Design review of the part built by this model. Coordinates are the model's own, in mm. A direction names the side the tool comes from. Give positions to 0.01 mm unless a question says otherwise; leave off trailing zeros. Loops run counter-clockwise (first coordinate to the right, second up) from the corner with the lowest first, then second, coordinate; pieces in that order, holes last. Notation, with made-up numbers: M 82.25,-10 L 91.25,-10 A18 cw 91.25,18 Z; hole C 2.5,48 d9. An arc over 180 degrees is marked long. Answer as CSV lines item,"result".
```python
from build123d import *

# Parameters (mm, degrees)
TABAN_FLAN_1_DEPTH         = 40
KES_EKSTR_ZYON1_DEPTH      = 1384.891767514
KES_EKSTR_ZYON1_DEPTH_BACK = 1384.891767514
IZIM2_W                    = 535
IZIM2_H                    = 265
KES_EKSTR_ZYON2_DEPTH      = 1384.891767514
KES_EKSTR_ZYON2_DEPTH_BACK = 1384.891767514
IZIM3_W                    = 1575
IZIM3_H                    = 360
KES_EKSTR_ZYON3_DEPTH      = 1384.891767514
KES_EKSTR_ZYON3_DEPTH_BACK = 1384.891767514
IZIM5_W                    = 535
IZIM5_H                    = 2


# Sheet-metal steps are written as plain solids
with BuildPart() as part:
    # Çizim1 → Taban-Flanş1 (new body)
    with BuildSketch(Plane.XY):
        Polygon((-517.241071282, 843.539135514), (-517.241071282, -126.460864486), (1057.758928718, -126.460864486), (1057.758928718, -891.460864486), (-1052.241071282, -891.460864486), (-1052.241071282, 843.539135514), align=None)
    extrude(amount=-TABAN_FLAN_1_DEPTH)

    # Çizim2 → Kes-Ekstrüzyon1 (cut, two sides: drawn at the far end of the back side and taken through both)
    with BuildSketch(Plane.XY.offset(-KES_EKSTR_ZYON1_DEPTH_BACK)):
        with Locations((-784.741071282, 711.039135514)):
            Rectangle(IZIM2_W, IZIM2_H)
    extrude(amount=KES_EKSTR_ZYON1_DEPTH + KES_EKSTR_ZYON1_DEPTH_BACK, mode=Mode.SUBTRACT)

    # Çizim3 → Kes-Ekstrüzyon2 (cut, two sides: drawn at the far end of the back side and taken through both)
    with BuildSketch(Plane.XY.offset(-KES_EKSTR_ZYON2_DEPTH_BACK)):
        with Locations((270.258928718, -306.460864486)):
            Rectangle(IZIM3_W, IZIM3_H)
    extrude(amount=KES_EKSTR_ZYON2_DEPTH + KES_EKSTR_ZYON2_DEPTH_BACK, mode=Mode.SUBTRACT)

    # Çizim5 → Kes-Ekstrüzyon3 (cut, two sides: drawn at the far end of the back side and taken through both)
    with BuildSketch(Plane.XY.offset(-KES_EKSTR_ZYON3_DEPTH_BACK)):
        with Locations((-784.741071282, 577.539135514)):
            Rectangle(IZIM5_W, IZIM5_H)
    extrude(amount=KES_EKSTR_ZYON3_DEPTH + KES_EKSTR_ZYON3_DEPTH_BACK, mode=Mode.SUBTRACT)


solid = part.part
```
1. We need section A-A, the plane z = -6.5. Write out the cut boundary in (x, y), plus the area to 3 significant figures.
Answer block:
outline,"M -1052.24,-891.46 L 1057.76,-891.46 L 1057.76,-486.46 L -517.24,-486.46 L -517.24,576.54 L -1052.24,576.54 Z"
area,"1,420,000 mm²"
2. For faces 1 (the flat face through (-788, 576.539, -20)), 2 (the flat face through (259, -486.461, -20)), list the 3-axis set-ups (+Z, -Z, +X, -X, +Y, -Y) from which the entire face can be reached by the end or side of a thin tool; tool diameter is ignored.
Answer block:
face 1,"+Z, -Z, +X, -X, +Y"
face 2,"+Z, -Z, +X, +Y"
3. We need section C-C, the plane x = 741.5. Write out the cut boundary in (y, z).
Answer block:
outline,"M -891.46,-40 L -486.46,-40 L -486.46,0 L -891.46,0 Z"
4. We need section B-B, the plane y = -316.5. Write out the cut boundary in (x, z), plus the area to 3 significant figures.
Answer block:
outline,"M -1052.24,-40 L -517.24,-40 L -517.24,0 L -1052.24,0 Z"
area,"21,400 mm²"
5. To check wall thickness, follow L1, parallel to X at y = 375.5, z = -12.5; L2, parallel to Y at x = -312.5, z = -5. State the ranges of each line that lie inside material, in increasing order. Write a range as [from, to].
Answer block:
L1,"[-1052.24, -517.24]"
L2,"[-891.46, -486.46]"
6. For P1, Ø1, axis at y = -259, z = -13, coming from the +X side; P2, Ø20, axis at x = 167.5, z = -16.5, coming from the +Y side, all flat-tipped, find the tip position at first contact; note any pin that passes through.
Answer block:
P1,"x = -517.24"
P2,"y = -486.46"
